Check sheet for the modelled part. Datum: model origin and axes. Units: mm. Face numbers are marked on the shaded views. A direction names the side the tool comes from. Give positions to 0.01 mm unless a question says otherwise; leave off trailing zeros. Order: outer loops, then holes, each group sorted by start corner. A loop starts at its lowest first (then second) coordinate and runs counter-clockwise, first axis right, second up.
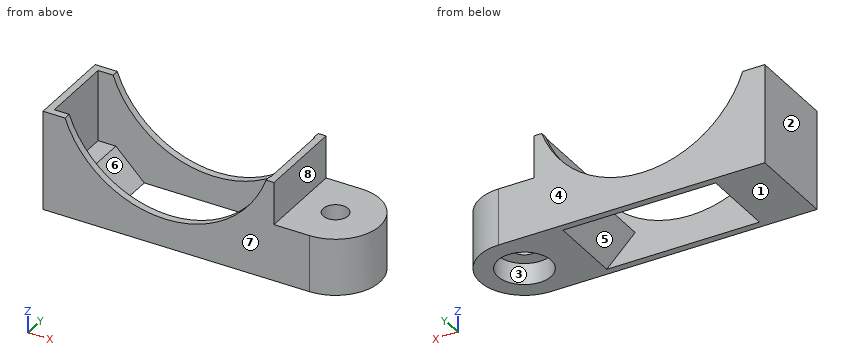
```python
from build123d import *

# Parameters (mm, degrees)
F0_R     = 1.75
F1_DEPTH = 8
F0_W     = 32.5
F0_H     = 12.5
F2_DEPTH = 14
F0_W_2   = 6.5
F0_H_2   = 10.5
F3_DEPTH = 4
F4_SIZE  = 3.99999
F6_DEPTH = 25
F7_R     = 3.75
F7_R_2   = 1.75
F8_DEPTH = 3


# Not quite as in the source:
# - a fillet or chamfer is up to 0.001 mm smaller than in the source, because OpenCascade refuses the exact size


with BuildPart() as f1:
    # F0 (on Top) → F1 (new body)
    with BuildSketch(Plane.XY):
        with BuildLine():
            Line((16.25, 6.25), (16.25, -6.25))
            Line((16.25, -6.25), (21.25, -6.25))
            ThreePointArc((21.25, -6.25), (27.5, 0), (21.25, 6.25))
            Line((21.25, 6.25), (16.25, 6.25))
        make_face()
        with Locations((21.25, 0)):
            Circle(F0_R, mode=Mode.SUBTRACT)
    extrude(amount=F1_DEPTH)

    # F0 (on Top) → F2 (join)
    with BuildSketch(Plane.XY):
        Rectangle(F0_W, F0_H)
        Polygon((15.25, 5.25), (15.25, -5.25), (8.75, -5.25), (-8.75, -5.25), (-15.25, -5.25), (-15.25, 5.25), (-8.75, 5.25), (8.75, 5.25), align=None, mode=Mode.SUBTRACT)
    extrude(amount=F2_DEPTH)

    # F0 (on Top) → F3 (join)
    with BuildSketch(Plane.XY):
        with Locations((12, 0)):
            Rectangle(F0_W_2, F0_H_2)
        with Locations((-12, 0)):
            Rectangle(F0_W_2, F0_H_2)
    extrude(amount=F3_DEPTH)

    # F4 (size 4 in the source; OpenCascade refuses exactly that, so slightly less here)
    f4_edges = [f1.edges().sort_by_distance(p)[0] for p in [
        (-8.75, 0, 4),
        (8.75, 0, 0),
    ]]
    chamfer(f4_edges, length=F4_SIZE)

    # F5 (on face) → F6 (cut)
    with BuildSketch(Plane.XZ.offset(6.25)):
        with BuildLine():
            Line((15.1421356237, 14), (-13.1421356237, 14))
            ThreePointArc((-13.1421356237, 14), (1, 4), (15.1421356237, 14))
        make_face()
    extrude(amount=-F6_DEPTH, mode=Mode.SUBTRACT)

    # F7 (on face) → F8 (cut)
    with BuildSketch(Plane.XY):
        with Locations((21.25, 0)):
            Circle(F7_R)
        with Locations((21.25, 0)):
            Circle(F7_R_2, mode=Mode.SUBTRACT)
    extrude(amount=F8_DEPTH, mode=Mode.SUBTRACT)


solid = f1.part
```
Q1. Sectioned sample at C-C, the plane z = 4.5. Record the cut outline in (x, y), plus the area to 3 significant figures.
Q2. Sectioned sample at A-A, the plane y = 0. Count the separate pieces of the cut face and the enclosed holes in it, plus the area to 3 significant figures.
Q3. Sectioned sample at D-D, the plane z = 11. Record the cut outline in (x, y), plus the area to 3 significant figures.
Q4. Draft check along X on the marked faces 1, 2 and 3. Enter one of: pulls with the +X half, pulls with the -X half, needs draft (parallel to the pull), parting line crosses it, or undercut.
Q5. Go/stop test with flat-tipped pins: P1, Ø6, axis at x = 21.25, y = 0, coming from the +Z side; P2, Ø6.5, axis at y = 1, z = 12, coming from the +X side; P3, Ø2, axis at y = 2.5, z = 2.5, coming from the +X side. Record where each tip stops, or that it passes through.
Q6. Tool access check on the marked faces 4, 5, 6, 7 and 8. Record the directions out of +Z, -Z, +X, -X, +Y, -Y that give a thin tool (end or side, any length) a straight path to the whole face; none if there is none.
Q7. Sectioned sample at B-B, the plane x = -8. Record the cut outline in (y, z).
Q8. Material ranges on line 1 (Y direction, x = 21.25, z = 4.8); line 2 (X direction, y = -0.75, z = 10.75); line 3 (X direction, y = -0.75, z = 6.75), recorded low to high.
Filled in:
1. outline: (-16.25, -6.25) - (-2.84, -6.25) - (-2.84, -5.25) - (-15.25, -5.25) - (-15.25, 5.25) - (-2.84, 5.25) - (-2.84, 6.25) - (-16.25, 6.25) - close; (4.84, -6.25) - (21.25, -6.25) arc R6.25 ccw to (21.25, 6.25) - (4.84, 6.25) - (4.84, 5.25) - (15.25, 5.25) - (15.25, -5.25) - (4.84, -5.25) - close; hole circle Ø3.5 at (21.25, 0)
1. area: 185 mm2
2. separate pieces: 3
2. enclosed holes: 0
2. area: 114 mm2
3. outline: (-16.25, -6.25) - (-11.69, -6.25) - (-11.69, -5.25) - (-15.25, -5.25) - (-15.25, 5.25) - (-11.69, 5.25) - (-11.69, 6.25) - (-16.25, 6.25) - close; (13.69, -6.25) - (16.25, -6.25) - (16.25, 6.25) - (13.69, 6.25) - (13.69, 5.25) - (15.25, 5.25) - (15.25, -5.25) - (13.69, -5.25) - close
3. area: 35.2 mm2
4. face 1: needs draft
4. face 2: pulls with the -X half
4. face 3: undercut
5. P1: stops at z = 8
5. P2: stops at x = 16.25
5. P3: stops at x = 27.32
6. face 4: +Z, -Z, +X, -X, +Y
6. face 5: -Z
6. face 6: +Z
6. face 7: +Z, -Z, +X, -X, -Y
6. face 8: +Z, +X, +Y, -Y
7. outline: (-6.25, 0) - (-5.25, 0) - (-5.25, 7) - (-6.25, 7) - close; (5.25, 0) - (6.25, 0) - (6.25, 7) - (5.25, 7) - close
8. line 1: y = -6.25 to -1.75, 1.75 to 6.25
8. line 2: x = -16.25 to -15.25, 15.25 to 16.25
8. line 3: x = -16.25 to -15.25, 15.25 to 19.67, 22.83 to 27.45
